The listing builds one solid part. Answer for the finished solid, in the listing's coordinates (mm). A direction names the side the tool comes from. Give positions to 0.01 mm unless a question says otherwise; leave off trailing zeros. Order: outer loops, then holes, each group sorted by start corner. A loop starts at its lowest first (then second) coordinate and runs counter-clockwise, first axis right, second up. Notation, with made-up numbers: (6.5, 65.5) - (14.5, 65.5) arc R37 ccw to (14.5, 102.5) - close; hole circle Ø6 at (62, 20). An arc over 180 degrees is marked (long way). Answer as a JSON object with one key per item and string values. Group by question number.
Q1. A cutting plane is placed at D-D, the plane x = -76.5. Give the vertices of the cut face in (y, z), and give its area (3 significant figures).
Q2. A cutting plane is placed at C-C, the plane x = -57.5. Give the vertices of the cut face in (y, z).
Q3. A cutting plane is placed at B-B, the plane z = 8.5. Give the vertices of the cut face in (x, y).
Q4. Given pin 1 (3 mm diameter, centred on x = 4.5, z = 2.5, fed in from -Y); pin 2 (2.5 mm diameter, centred on y = 32.5, z = 20, fed in from -X); pin 3 (5 mm diameter, centred on x = 70.5, z = 13, fed in from +Y); pin 4 (8.5 mm diameter, centred on x = 21, z = 11, fed in from -Y), each flat-ended and moving along its own axis, determine where each tip first touches the part or whether it passes through.
Q5. A cutting plane is placed at A-A, the plane y = -8.5. Give the vertices of the cut face in (x, z).
Q6. The mould has two halves that part along Y. Classify faces 1 (the face through (-32, 37.403, 2)), 2 (the face through (0.8, -21.597, 27.3)), 3 (the face through (-0.5, -24.097, 31.6)): released by +Y, released by -Y, zero draft, split by the parting line, or undercut.
Q7. For faces 4 (the face through (72.675, 11, 3)), 5 (the face through (32.175, -24, 2)), 6 (the face through (71, -19.61, 16)), 7 (the face through (74, -11, 0.357)), 8 (the face through (36.175, -24, 2)), determine the directions among +Z, -Z, +X, -X, +Y, -Y from which every point of the face is accessible in a straight line to the end or side of a thin tool.
Q8. Consider line 1 (X direction, y = -16.5, z = 32); line 2 (X direction, y = 33, z = 24); line 3 (Z direction, x = -52, y = 31). Determine where each line is inside the solid, lowest interval first.
from build123d import *

# Parameters (mm, degrees)
SKETCH1_W               = 150
SKETCH1_H               = 55
SKETCH1_W_2             = 143
SKETCH1_H_2             = 50
BOSS_EXTRUDE1_DEPTH     = 30
CUT_EXTRUDE6_DEPTH      = 46
CUT_EXTRUDE6_DEPTH_BACK = 1
SKETCH2_W               = 170
SKETCH2_H               = 60
SKETCH3_W               = 176.272583165
SKETCH3_H               = 65
BOSS_EXTRUDE3_DEPTH     = 12
SKETCH4_W               = 170
SKETCH4_H               = 60
CUT_EXTRUDE7_DEPTH      = 10
CUT_EXTRUDE8_DEPTH      = 102.484371807
CUT_EXTRUDE8_DEPTH_BACK = 102.484371807
SKETCH5_W               = 143
SKETCH5_H               = 50
SKETCH6_W               = 4
SKETCH6_H               = 4
BOSS_EXTRUDE5_DEPTH     = 4
CUT_EXTRUDE9_DEPTH      = 105.971794883
CUT_EXTRUDE9_DEPTH_BACK = 4
SKETCH7_R               = 1
SKETCH8_W               = 28
SKETCH8_H               = 17
CUT_EXTRUDE12_DEPTH     = 10
SKETCH9_W               = 130
SKETCH9_H               = 23.050427834
CUT_EXTRUDE13_DEPTH     = 72
SKETCH10_W              = 20
SKETCH10_H              = 50.513415504
CUT_EXTRUDE14_DEPTH     = 177
SKETCH11_W              = 160
SKETCH11_H              = 10.657938717
CUT_EXTRUDE15_DEPTH     = 177


with BuildPart() as part:
    # Sketch1 → Boss-Extrude1 (new body)
    with BuildSketch(Plane.XY):
        with Locations((1.175180371, 5.902996071)):
            Rectangle(SKETCH1_W, SKETCH1_H)
        with Locations((1.175180371, 5.902996071)):
            Rectangle(SKETCH1_W_2, SKETCH1_H_2, mode=Mode.SUBTRACT)
    extrude(amount=BOSS_EXTRUDE1_DEPTH)

    # Sketch2 → Cut-Extrude6 (cut, two sides: drawn at the far end of the back side and taken through both)
    with BuildSketch(Plane.XY.offset(30).offset(-CUT_EXTRUDE6_DEPTH_BACK)):
        with Locations((1.175180371, 5.902996071)):
            Rectangle(SKETCH2_W, SKETCH2_H)
    extrude(amount=CUT_EXTRUDE6_DEPTH + CUT_EXTRUDE6_DEPTH_BACK, mode=Mode.SUBTRACT)

    # Sketch3 → Boss-Extrude3 (add)
    with BuildSketch(Plane.XY.offset(29)):
        with Locations((0.538888789, 5.902996071)):
            Rectangle(SKETCH3_W, SKETCH3_H)
    extrude(amount=BOSS_EXTRUDE3_DEPTH)

    # Sketch4 → Cut-Extrude7 (cut)
    with BuildSketch(Plane.XY.offset(41)):
        with Locations((-0.097402794, 5.902996071)):
            Rectangle(SKETCH4_W, SKETCH4_H)
    extrude(amount=-CUT_EXTRUDE7_DEPTH, mode=Mode.SUBTRACT)

    # Sketch5 → Cut-Extrude8 (cut, two sides: drawn at the far end of the back side and taken through both)
    with BuildSketch(Plane.XY.offset(31).offset(-CUT_EXTRUDE8_DEPTH_BACK)):
        with Locations((1.175180371, 5.902996071)):
            Rectangle(SKETCH5_W, SKETCH5_H)
    extrude(amount=CUT_EXTRUDE8_DEPTH + CUT_EXTRUDE8_DEPTH_BACK, mode=Mode.SUBTRACT)

    # Sketch6 → Boss-Extrude5 (add)
    with BuildSketch(Plane(origin=(0, 0, 0), x_dir=(-1, 0, 0), z_dir=(0, 0, -1))):
        with Locations((-34.175180371, -23.597003929)):
            Rectangle(SKETCH6_W, SKETCH6_H)
        with Locations((31.824819629, -23.597003929)):
            Rectangle(SKETCH6_W, SKETCH6_H)
        with Locations((-34.175180371, 35.402996071)):
            Rectangle(SKETCH6_W, SKETCH6_H)
        with Locations((31.824819629, 35.402996071)):
            Rectangle(SKETCH6_W, SKETCH6_H)
    extrude(amount=-BOSS_EXTRUDE5_DEPTH)

    # Sketch7 → Cut-Extrude9 (cut, two sides: drawn at the far end of the back side and taken through both)
    with BuildSketch(Plane(origin=(0, 0, 0), x_dir=(-1, 0, 0), z_dir=(0, 0, -1)).offset(-CUT_EXTRUDE9_DEPTH_BACK)):
        with Locations(Location((-34.175180371, 35.402996071, 0), (0, 0, 180))):
            Circle(SKETCH7_R)
        with Locations(Location((31.824819629, 35.402996071, 0), (0, 0, 180))):
            Circle(SKETCH7_R)
        with Locations(Location((31.824819629, -23.597003929, 0), (0, 0, 180))):
            Circle(SKETCH7_R)
        with Locations(Location((-34.175180371, -23.597003929, 0), (0, 0, 180))):
            Circle(SKETCH7_R)
    extrude(amount=CUT_EXTRUDE9_DEPTH + CUT_EXTRUDE9_DEPTH_BACK, mode=Mode.SUBTRACT)

    # Sketch8 → Cut-Extrude12 (cut)
    with BuildSketch(Plane(origin=(76.175180371, 0, 0), x_dir=(0, 0, -1), z_dir=(1, 0, 0))):
        with Locations((-14.356573147, -10.597003929)):
            Rectangle(SKETCH8_W, SKETCH8_H)
    extrude(amount=-CUT_EXTRUDE12_DEPTH, mode=Mode.SUBTRACT)

    # Sketch9 → Cut-Extrude13 (cut)
    with BuildSketch(Plane(origin=(0, 33.402996071, 0), x_dir=(1, 0, 0), z_dir=(0, 1, 0))):
        with Locations((1.175180371, -15.525213917)):
            Rectangle(SKETCH9_W, SKETCH9_H)
    extrude(amount=-CUT_EXTRUDE13_DEPTH, mode=Mode.SUBTRACT)

    # Sketch10 → Cut-Extrude14 (cut)
    with BuildSketch(Plane.ZY.offset(73.824819629)):
        with Locations((16.5, 5.646288319)):
            Rectangle(SKETCH10_W, SKETCH10_H)
    extrude(amount=-CUT_EXTRUDE14_DEPTH, mode=Mode.SUBTRACT)

    # Sketch11 → Cut-Extrude15 (cut)
    with BuildSketch(Plane(origin=(0, 38.402996071, 0), x_dir=(1, 0, 0), z_dir=(0, 1, 0))):
        with Locations((0.675180371, -37.197220061)):
            Rectangle(SKETCH11_W, SKETCH11_H)
    extrude(amount=-CUT_EXTRUDE15_DEPTH, mode=Mode.SUBTRACT)


solid = part.part
Reply:
{
 "1": {"outline": "(-26.6, 29) - (38.4, 29) - (38.4, 31.87) - (35.9, 31.87) - (35.9, 31) - (-24.1, 31) - (-24.1, 31.87) - (-26.6, 31.87) - close", "area": "134 mm^2"},
 "2": {"outline": "(-26.6, 29) - (-21.6, 29) - (-21.6, 27.05) - (-19.1, 27.05) - (-19.1, 31) - (-24.1, 31) - (-24.1, 31.87) - (-26.6, 31.87) - close; (-21.6, 0) - (-19.1, 0) - (-19.1, 4) - (-21.6, 4) - close; (30.9, 0) - (33.4, 0) - (33.4, 4) - (30.9, 4) - close; (30.9, 27.05) - (33.4, 27.05) - (33.4, 29) - (38.4, 29) - (38.4, 31.87) - (35.9, 31.87) - (35.9, 31) - (30.9, 31) - close"},
 "3": {"outline": "(-73.82, -21.6) - (-63.82, -21.6) - (-63.82, -19.61) - (-73.82, -19.61) - close; (-73.82, 30.9) - (-63.82, 30.9) - (-63.82, 33.4) - (-73.82, 33.4) - close; (66.18, -21.6) - (76.18, -21.6) - (76.18, -19.61) - (66.18, -19.61) - close; (66.18, 30.9) - (76.18, 30.9) - (76.18, 33.4) - (66.18, 33.4) - close"},
 "4": {"pin 1": "stops at y = -21.6", "pin 2": "stops at x = -73.82", "pin 3": "stops at y = 33.4", "pin 4": "passes through"},
 "5": {"outline": "(-87.6, 29) - (-73.82, 29) - (-73.82, 26.5) - (-70.32, 26.5) - (-70.32, 31) - (-85.1, 31) - (-85.1, 41) - (-87.6, 41) - close; (-73.82, 0) - (-70.32, 0) - (-70.32, 6.5) - (-73.82, 6.5) - close; (72.68, 0) - (76.18, 0) - (76.18, 0.36) - (72.68, 0.36) - close; (72.68, 28.36) - (76.18, 28.36) - (76.18, 29) - (88.68, 29) - (88.68, 41) - (84.9, 41) - (84.9, 31) - (72.68, 31) - close"},
 "6": {"face 1": "released by +Y", "face 2": "released by -Y", "face 3": "undercut"},
 "7": {"face 4": "+Z, -Z", "face 5": "-Z, -Y", "face 6": "+X, -X", "face 7": "+X", "face 8": "-Z, +X, -Y"},
 "8": {"line 1": "x = -87.6 to -85.1, 84.9 to 88.68", "line 2": "x = -73.82 to -63.82, 66.18 to 76.18", "line 3": "z = 0 to 4, 27.05 to 31"}
}
